Design review of the part built by this model. Coordinates are the model's own, in mm. A direction names the side the tool comes from. Round coordinates to 2 decimals unless told otherwise and drop trailing zeros. Order: outer loops, then holes, each group sorted by start corner. A loop starts at its lowest first (then second) coordinate and runs counter-clockwise, first axis right, second up. Notation, with made-up numbers: (-34, 13) - (-29, 13) arc R20 cw to (-29, 29) - close; hole circle Ø6 at (-6, -21.5). An arc over 180 degrees is marked (long way). Use CSV: the item, a comma, the result in double quotes.
Autodesk Inventor part; units mm, degrees
ref_plane "YZ Plane" through (0, 0, 0) normal (1, 0, 0) x (0, 1, 0)
ref_plane "XZ Plane" through (0, 0, 0) normal (0, 1, 0) x (-1, 0, 0)
ref_plane "XY Plane" through (0, 0, 0) normal (0, 0, 1) x (1, 0, 0)
sketch "Sketch1" plane through (0, 0, 0) normal (0, 0, 1) x (1, 0, 0)
  circle A0 centre (0, 0) radius 0.925
  line L0 (5, 2.6) -> (-0.4566, 3.4576)
  arc A1 (-0.4566, 3.4576) -> (-0.4566, -3.4576) centre (-1, 0) ccw
  line L1 (-0.4566, -3.4576) -> (5, -2.6)
  line L2 (0, 0) -> (26, 0) construction
  line L3 (5, 2.6) -> (8, 2.6)
  arc A2 (8, -2.6) -> (8, 2.6) centre (8, 0) ccw
  line L4 (8, -2.6) -> (5, -2.6)
  dimension "d0" = 1.85
  dimension "d7" = 3.5
  dimension "d8" = 1
  dimension "d10" = 2.6
  dimension "d11" = 8
  dimension "d12" = 6
extrude "Extrusion1" add sketch "Sketch1" along normal blind 3
properties part number "slider_link_p5"
1) We need section D-D (x = 9.5). Give the boundary of the cut face in (y, z).
Data:
outline,"(-2.12, 0) - (2.12, 0) - (2.12, 3) - (-2.12, 3) - close"
2) For faces 1 (the face through (10.6, 0.1, 1.5)), 2 (the face through (7, -2.6, 1)), 3 (the face through (6, 2.6, 1)), list the 3-axis set-ups (+Z, -Z, +X, -X, +Y, -Y) from which the entire face can be reached by the end or side of a thin tool; tool diameter is ignored.
Data:
face 1,"+Z, -Z, +X"
face 2,"+Z, -Z, +X, -Y"
face 3,"+Z, -Z, +X, +Y"
3) To check wall thickness, follow L1, parallel to Y at x = 6.25, z = 2.15; L2, parallel to X at y = 0.5, z = 1.9; L3, parallel to Y at x = 0, z = 2.6 (3 decimals). State the ranges of each line that lie inside material, in increasing order. Write a range as from..to.
Data:
L1,"y = -2.6..2.6"
L2,"x = -4.46..-0.78, 0.78..10.55"
L3,"y = -3.386..-0.925, 0.925..3.386"
4) We need section B-B (z = 1.7). Give the boundary of the cut face in (x, y) (3 decimals), then the cut area to 3 significant figures.
Data:
outline,"(-0.457, -3.458) - (5, -2.6) - (8, -2.6) arc R2.6 ccw to (8, 2.6) - (5, 2.6) - (-0.457, 3.458) arc R3.5 ccw (long way) to start; hole circle Ø1.85 at (0, 0)"
area,"79.6 mm2"
5) We need section C-C (x = 0). Give the boundary of the cut face in (y, z) (3 decimals), then the cut area to 3 significant figures.
Data:
outline,"(-3.386, 0) - (-0.925, 0) - (-0.925, 3) - (-3.386, 3) - close; (0.925, 0) - (3.386, 0) - (3.386, 3) - (0.925, 3) - close"
area,"14.8 mm2"
6) We need section A-A (y = 0). Give the boundary of the cut face in (x, z) (3 decimals), then the cut area to 3 significant figures.
Data:
outline,"(-4.5, 0) - (-0.925, 0) - (-0.925, 3) - (-4.5, 3) - close; (0.925, 0) - (10.6, 0) - (10.6, 3) - (0.925, 3) - close"
area,"39.8 mm2"
7) The part is to be moulded in two halves that separate along X. For faces 4 (the face through (-0.201, 0.903, 1.479)), 5 (the face through (2.31, 3.023, 1.479)), 6 (the face through (3, 0, 0)), say which applies: +X half, -X half, draft (parallel to the pull), parting line (faces both ways), or undercut.
Data:
face 4,"undercut"
face 5,"+X half"
face 6,"draft"
8) Insertion check: pin 1 Ø0.9 at (x, z) = (6.5, 1) entering from +Y. The pin has a flat end and moves straight along its axis. Give the tip position at first contact, or say it passes through.
Data:
pin 1,"stops at y = 2.6"
